Print and shaded views of the part. All mm, measured from the part's lowest x, y and z. Round coordinates to 2 decimals unless told otherwise and drop trailing zeros. Loops run counter-clockwise (first coordinate to the right, second up) from the corner with the lowest first, then second, coordinate; pieces in that order, holes last. Notation, with made-up numbers: (69.5, -23.5) -> (127.5, -23.5) arc R24 cw to (127.5, 12.5) -> close; hole circle Ø1 at (17.5, 68.5). An arc over 180 degrees is marked (long way). Use a Markdown table: item, result.
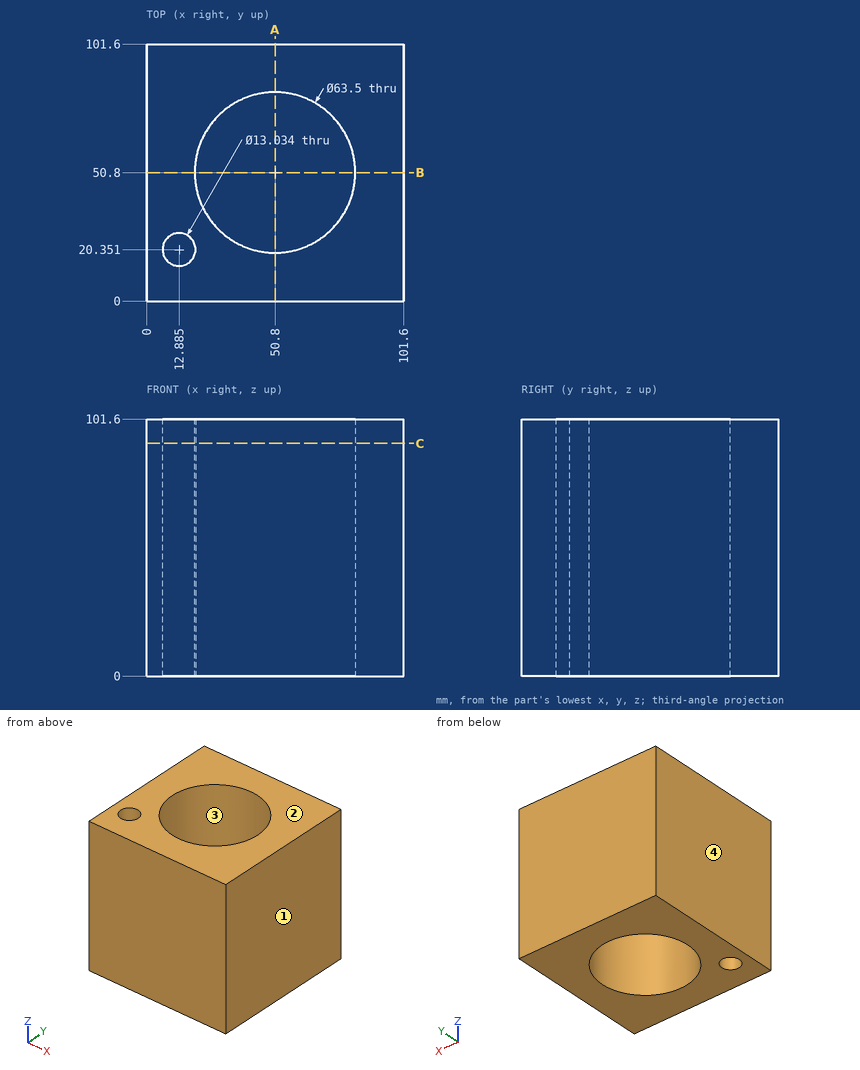
Q1. Band-saw the part on C-C, the plane z = 92. Give the number of separate pieces and of enclosed holes in the cut face, plus the area to 3 significant figures.
Results list:
| item | result |
|---|---|
| separate pieces | 1 |
| enclosed holes | 2 |
| area | 7,020 mm² |
Q2. Drill centre lines: L1, parallel to Y at x = 52, z = 89; L2, parallel to Y at x = 13, z = 87 (1 decimal); L3, parallel to X at y = 35.5, z = 60. Where is each one in solid material? Low to high. Write a range as from..to.
Results list:
| item | result |
|---|---|
| L1 | y = 0..19.07, 82.53..101.6 |
| L2 | y = 0..13.8, 26.9..101.6 |
| L3 | x = 0..22.98, 78.62..101.6 |
Q3. Pull direction X, two halves, no side cores. Call the marked faces 1, 2, 3 and 4: released by +X, released by -X, zero draft, split by the parting line, or undercut.
Results list:
| item | result |
|---|---|
| face 1 | released by +X |
| face 2 | zero draft |
| face 3 | undercut |
| face 4 | released by -X |
Q4. Flat gauge pins, fed straight in: pin 1 (6 mm diameter, centred on x = 88, y = 52, fed in from -Z); pin 2 (10.5 mm diameter, centred on x = 12.89, y = 20.35, fed in from -Z). Where does each tip first touch, or does it go through?
Results list:
| item | result |
|---|---|
| pin 1 | stops at z = 0 |
| pin 2 | passes through |
Q5. Band-saw the part on A-A, the plane x = 50.8. Give the cut face in (y, z), plus the area to 3 significant figures.
Results list:
| item | result |
|---|---|
| outline | (0, 0) -> (19.05, 0) -> (19.05, 101.6) -> (0, 101.6) -> close; (82.55, 0) -> (101.6, 0) -> (101.6, 101.6) -> (82.55, 101.6) -> close |
| area | 3,870 mm² |
